Part model, mm, in its own coordinate system. A direction names the side the tool comes from. Round coordinates to 2 decimals unless told otherwise and drop trailing zeros. Write each loop counter-clockwise with the first axis right and the second up, starting at its lowest first coordinate (ties: lowest second). Pieces come first, ordered by that corner, then holes. Notation, with made-up numbers: M 63,-22.75 L 110,-22.75 A18 ccw 110,-14.75 Z; hole C 30,88.25 d1. An arc over 180 degrees is marked long. One line per question, with ' | ' between items. Start each with the question number.
1) Saw through at C-C (y = 26). List the corners of the cut face in (x, z).
2) Saw through at B-B (z = -1.7). List the corners of the cut face in (x, y), plus the area to 3 significant figures.
3) Mould opens along Y. For faces 1 (the face through (1, 0, -2.54)), 2 (the face through (34.604, 28.398, -1.295)), 3 (the face through (1, -33.274, -4)) say: pulls with the +Y half, pulls with the -Y half, needs draft (parallel to the pull), parting line crosses it, or undercut.
4) Drop flat-ended pins along their axis: pin 1 Ø2 at (x, y) = (-35.56, 26.9) entering from -Z; pin 2 Ø3.5 at (x, y) = (-36, 28) entering from -Z; pin 3 Ø6 at (x, y) = (-10, -12.5) entering from +Z; pin 4 Ø4.5 at (x, y) = (-35.56, 26.9) entering from +Z. Give the stop position or say it passes through.
5) Tool access for faces 4 (the face through (-33.033, 24.581, -0.995)), 5 (the face through (-37, 25, 0.508)), 6 (the face through (-36, 29, -3.048)): list every direction of +Z, -Z, +X, -X, +Y, -Y with a clear straight run to the whole face (end or side of a thin tool).
6) Saw through at A-A (x = 35.56). List the corners of the cut face in (y, z), plus the area to 3 significant figures.
7) Saw through at D-D (x = -1.5). List the corners of the cut face in (y, z), plus the area to 3 significant figures.
8) Wall check: probe 1 along Y at (x, z) = (35.56, -4.2); probe 2 along X at (y, z) = (27, -4.5); probe 3 along Y at (x, z) = (35.56, -1.5). Give the ranges that are in metal, low to high. Write a range as [from, to].
Solid Edge part; units mm, degrees
sketch "Sketch1" plane through (0, 2.54, -2.54) normal (0, 0, -1) x (-1, 0, 0)
  line L0 (-41.529, 29.21) -> (-41.529, -34.29)
  arc A0 (-41.529, -34.29) -> (-40.005, -35.814) centre (-40.005, -34.29) ccw
  line L1 (-40.005, -35.814) -> (40.005, -35.814)
  arc A1 (40.005, -35.814) -> (41.529, -34.29) centre (40.005, -34.29) ccw
  line L2 (41.529, -34.29) -> (41.529, 29.21)
  arc A2 (41.529, 29.21) -> (40.005, 30.734) centre (40.005, 29.21) ccw
  line L3 (40.005, 30.734) -> (-40.005, 30.734)
  arc A3 (-40.005, 30.734) -> (-41.529, 29.21) centre (-40.005, 29.21) ccw
extrude "Protrusion1" add sketch "Sketch1" along normal blind 2.54
sketch "Sketch2" plane through (36.703, 28.2448, 0.508) normal (0, 0, -1) x (-1, 0, 0)
  circle A0 centre (72.263, -1.3462) radius 3.429
  circle A1 centre (1.143, -1.3462) radius 3.429
extrude "ExtrudedProtrusion_2" add sketch "Sketch2" along normal up to next
sketch "Sketch3" plane through (0, 0, -5.08) normal (0, 0, -1) x (-1, 0, 0)
  circle A0 centre (-35.56, 26.8986) radius 1.778
  circle A1 centre (35.56, 26.8986) radius 1.778
extrude "Cutout1" cut sketch "Sketch3" against normal up to next
sketch "Sketch4" plane through (0, 0, -5.08) normal (0, 0, -1) x (-1, 0, 0)
  circle A0 centre (-35.56, 26.8986) radius 3.556
  circle A1 centre (35.56, 26.8986) radius 3.556
extrude "ExtrudedCutout_2" cut sketch "Sketch4" against normal blind 2.032
fillet "Round_1" [suppressed]
Answer key:
1) outline: M -41.53,-5.08 L -39,-5.08 L -39,-3.05 L -37.09,-3.05 L -37.09,0.51 L -38.87,0.51 L -38.87,-2.54 L -41.53,-2.54 Z; M -34.03,-3.05 L -32.12,-3.05 L -32.12,-5.08 L 32.12,-5.08 L 32.12,-3.05 L 34.03,-3.05 L 34.03,0.51 L 32.25,0.51 L 32.25,-2.54 L -32.25,-2.54 L -32.25,0.51 L -34.03,0.51 Z; M 37.09,-3.05 L 39,-3.05 L 39,-5.08 L 41.53,-5.08 L 41.53,-2.54 L 38.87,-2.54 L 38.87,0.51 L 37.09,0.51 Z
2) outline: C -35.56,26.9 d6.86; C 35.56,26.9 d6.86; hole C -35.56,26.9 d3.56; hole C 35.56,26.9 d3.56 | area: 54.0 mm2
3) face 1: needs draft | face 2: undercut | face 3: pulls with the -Y half
4) pin 1: passes through | pin 2: stops at z = -3.05 | pin 3: stops at z = -2.54 | pin 4: stops at z = 0.51
5) face 4: +Z | face 5: +Z, +X, -X, +Y, -Y | face 6: -Z
6) outline: M -33.27,-5.08 L 23.34,-5.08 L 23.34,-3.05 L 25.12,-3.05 L 25.12,0.51 L 23.47,0.51 L 23.47,-2.54 L -33.27,-2.54 Z; M 28.68,-3.05 L 30.45,-3.05 L 30.45,-5.08 L 33.27,-5.08 L 33.27,-2.54 L 30.33,-2.54 L 30.33,0.51 L 28.68,0.51 Z | area: 163 mm2
7) outline: M -33.27,-5.08 L 33.27,-5.08 L 33.27,-2.54 L -33.27,-2.54 Z | area: 169 mm2
8) probe 1: y = [-33.27, 23.34], [30.45, 33.27] | probe 2: x = [-41.53, -39.11], [-32.01, 32.01], [39.11, 41.53] | probe 3: y = [23.47, 25.12], [28.68, 30.33]
